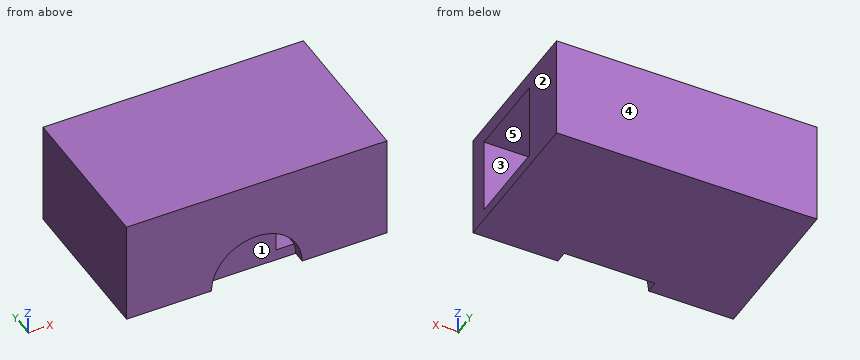
```python
from build123d import *

# Parameters (mm, degrees)
F0_W       = 261.3020315766
F0_H       = 159.2612788081
F1_DEPTH   = 105.156
F2_W       = 119.9641153216
F2_H       = 77.4333942682
F3_DEPTH   = 104.902
F5_DEPTH   = 63.5
F1_FACE2_W = 261.3020315766
F1_FACE2_H = 105.156
F7_DEPTH   = 51.308


with BuildPart() as f1:
    # F0 (on Top) → F1 (new body)
    with BuildSketch(Plane.XY):
        with Locations((-55.9731982648, 11.1682154238)):
            Rectangle(F0_W, F0_H)
    extrude(amount=F1_DEPTH)

    # F2 (on face) → F3 (cut)
    with BuildSketch(Plane.YZ.offset(74.6778175235)):
        with Locations((12.3364068568, 50.0526567921)):
            Rectangle(F2_W, F2_H)
    extrude(amount=-F3_DEPTH, mode=Mode.SUBTRACT)

    # F4 (on face) → F5 (cut)
    with BuildSketch(Plane.XZ.offset(68.4624239802)):
        with BuildLine():
            Line((-101.4091865089, 0), (-10.5372100208, 0))
            ThreePointArc((-10.5372100208, 0), (-55.9731982648, 45.435988244), (-101.4091865089, 0))
        make_face()
    extrude(amount=-F5_DEPTH, mode=Mode.SUBTRACT)

    # F6 (on face) + F1_face2 (on face) + F5_face (on face) → F7 (join)
    with BuildSketch(Plane(origin=(0, 90.7988548279, 0), x_dir=(-1, 0, 0), z_dir=(0, 1, 0))):
        with BuildLine():
            Line((4.3711580431, 0), (100.9396470988, 0))
            ThreePointArc((100.9396470988, 0), (52.655402571, 48.2842445279), (4.3711580431, 0))
        make_face()
    with BuildSketch(Plane(origin=(-55.9731982648, 90.7988548279, 52.578), x_dir=(-1, 0, 0), z_dir=(0, 1, 0))):
        Rectangle(F1_FACE2_W, F1_FACE2_H)
    with BuildSketch(Plane(origin=(-59.2987118698, -4.9624239802, 19.1021444838), x_dir=(1, 0, 0), z_dir=(0, -1, 0))):
        with BuildLine():
            ThreePointArc((29.0745293932, 18.3333629075), (-17.8227374937, 21.1120383773), (-42.1104746391, -19.1021444838))
            Line((-42.1104746391, -19.1021444838), (48.761501849, -19.1021444838))
            ThreePointArc((48.761501849, -19.1021444838), (48.4008605817, -13.388815976), (47.3246618506, -7.7661848257))
            Line((47.3246618506, -7.7661848257), (29.0745293932, -7.7661848257))
            Line((29.0745293932, -7.7661848257), (29.0745293932, 18.3333629075))
        make_face()
    extrude(amount=-F7_DEPTH, dir=(0, 1, 0))


solid = f1.part
```
Source: CAD feature listing. Evaluate the final solid. Frame: model axes, mm. Face numbers are marked on the shaded views. A direction names the side the tool comes from. Round coordinates to 2 decimals unless told otherwise and drop trailing zeros. Write each loop counter-clockwise with the first axis right and the second up, starting at its lowest first coordinate (ties: lowest second). Pieces come first, ordered by that corner, then holes. Notation, with made-up numbers: M 59,-35 L 81,-35 A26 cw 81,-16 Z; hole C 3.5,7.25 d10. An arc over 180 degrees is marked long. Use CSV: the item, a comma, the result in double quotes. Start each with the question number.
Q1. Cut plane C-C on y = -18. Output: boundary loops of the cut face in (x, z), plus the area to 3 significant figures.
Q2. Access query for the marked faces 4 and 5. Directions: +Z, -Z, +X, -X, +Y, -Y. A direction counts if a zero-diameter tool reaches every point of the face in a straight line with its end or side. Return the directions, or none.
Q3. Cut plane D-D on z = 57. Output: boundary loops of the cut face in (x, y), plus the area to 3 significant figures.
Q4. Pull-direction query (X, two-part tool) for the marked faces 1, 2 and 3; classes: +X half, -X half, draft (parallel to the pull), parting line (faces both ways), or undercut.
Q5. Cut plane A-A on x = 48.5. Output: boundary loops of the cut face in (y, z), plus the area to 3 significant figures.
Q6. Cut plane B-B on z = 34.5. Output: boundary loops of the cut face in (x, y), plus the area to 3 significant figures.
Q7. Line query: line 1 (Z direction, x = -22, y = -18); line 2 (Y direction, x = -26, z = 38); line 3 (X direction, y = 11.5, z = 69). Output: solid intervals per line, ascending. Write a range as from..to.
Q8. First-contact query: P1, Ø23, axis at y = -14.5, z = 60.5, coming from the +X side; P2, Ø13.5, axis at x = -59, z = 32.5, coming from the -Y side. Flat tips, straight axial feed; report the tip coordinate or a pass-through.
Results found:
1,outline,"M -186.62,0 L 74.68,0 L 74.68,11.34 L -30.22,11.34 L -30.22,88.77 L 74.68,88.77 L 74.68,105.16 L -186.62,105.16 Z"
1,area,"19,400 mm^2"
2,face 4,"+Z, -Z, +X, -X, +Y"
2,face 5,"+X"
3,outline,"M -186.62,-68.46 L 74.68,-68.46 L 74.68,-47.65 L -30.22,-47.65 L -30.22,39.49 L 74.68,39.49 L 74.68,90.8 L -186.62,90.8 Z"
3,area,"32,500 mm^2"
4,face 1,"undercut"
4,face 2,"+X half"
4,face 3,"draft"
5,outline,"M -68.46,0 L 90.8,0 L 90.8,105.16 L -68.46,105.16 Z; hole M -47.65,11.34 L 39.49,11.34 L 39.49,88.77 L -47.65,88.77 Z"
5,area,"10,000 mm^2"
6,outline,"M -186.62,-68.46 L -85.54,-68.46 L -85.54,-56.27 L -30.22,-56.27 L -30.22,39.49 L 74.68,39.49 L 74.68,90.8 L -186.62,90.8 Z; M -26.41,-68.46 L 74.68,-68.46 L 74.68,-47.65 L -26.41,-47.65 Z"
6,area,"31,700 mm^2"
7,line 1,"0..11.34, 88.77..105.16"
7,line 2,"-68.46..-47.65, 39.49..90.8"
7,line 3,"-186.62..-30.22"
8,P1,"x = -30.22"
8,P2,"y = -56.27"
